Verification items for the finished model (mm, model axes). Face numbers are marked on the shaded views. A direction names the side the tool comes from. Give positions to 0.01 mm unless a question says otherwise; leave off trailing zeros. Write each loop counter-clockwise with the first axis right and the second up, starting at its lowest first coordinate (ties: lowest second). Pieces come first, ordered by that corner, then holes.
from build123d import *

# Parameters (mm, degrees)
F0_R     = 6.5
F1_DEPTH = 8
F3_DEPTH = 4
F4_R     = 4
F5_DEPTH = 45
F6_R     = 4
F6_R_2   = 3.4
F7_DEPTH = 28
F8_SIZE  = 1


with BuildPart() as f1:
    # F0 (on Front) → F1 (new body)
    with BuildSketch(Plane.XZ):
        Circle(F0_R)
    extrude(amount=-F1_DEPTH)

    # F2 (on face) → F3 (cut)
    with BuildSketch(Plane.XZ):
        Polygon((3, 1.732051), (0, 3.464102), (-3, 1.732051), (-3, -1.732051), (0, -3.464102), (3, -1.732051), align=None)
    extrude(amount=-F3_DEPTH, mode=Mode.SUBTRACT)

    # F4 (on face) → F5 (join)
    with BuildSketch(Plane(origin=(0, 8, 0), x_dir=(-1, 0, 0), z_dir=(0, 1, 0))):
        Circle(F4_R)
    extrude(amount=F5_DEPTH)

    # F6 (on face) → F7 (cut)
    with BuildSketch(Plane(origin=(0, 53, 0), x_dir=(-1, 0, 0), z_dir=(0, 1, 0))):
        Circle(F6_R)
        Circle(F6_R_2, mode=Mode.SUBTRACT)
    extrude(amount=-F7_DEPTH, mode=Mode.SUBTRACT)

    # F8
    f8_edges = [f1.edges().sort_by_distance(p)[0] for p in [
        (-6.5, 0, 0),
    ]]
    chamfer(f8_edges, length=F8_SIZE)


solid = f1.part
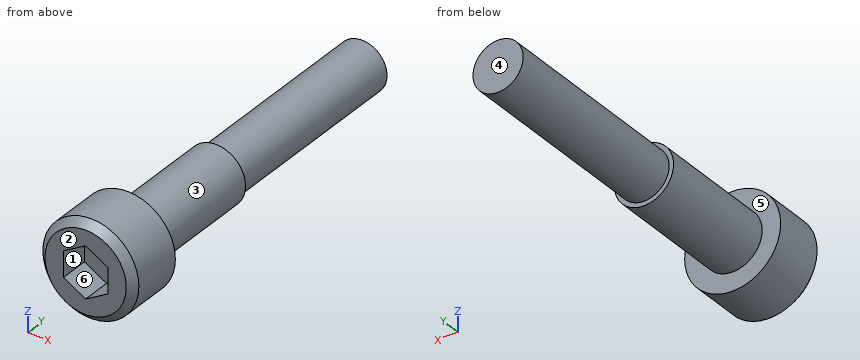
Item 1: Sectioned sample at B-B on z = 0. Record the cut outline in (x, y), then the cut area to 3 significant figures.
Answer key:
outline: (-6.5, 1) - (-5.5, 0) - (-3, 0) - (-3, 4) - (3, 4) - (3, 0) - (5.5, 0) - (6.5, 1) - (6.5, 8) - (4, 8) - (4, 25) - (3.4, 25) - (3.4, 53) - (-3.4, 53) - (-3.4, 25) - (-4, 25) - (-4, 8) - (-6.5, 8) - close
area: 405 mm2
Item 2: Set-up check for the marked faces 4, 5 and 6: record each of +Z, -Z, +X, -X, +Y, -Y from which the full face is reachable in a straight line by a thin tool's end or side.
Answer key:
face 4: +Z, -Z, +X, -X, +Y
face 5: +Y
face 6: -Y
Item 3: Sectioned sample at C-C on y = 48. Record the cut outline in (x, z).
Answer key:
outline: circle Ø6.8 at (0, 0)
Item 4: Release check for a two-part mould opening along X. For the marked faces 1, 2 and 3 record: released by +X, released by -X, zero draft, split by the parting line, or undercut.
Answer key:
face 1: undercut
face 2: zero draft
face 3: split by the parting line
Item 5: Scan lines: line 1 along Y through (x, z) = (-3.5, 0); line 2 along X through (y, z) = (16.5, -0.25); line 3 along X through (y, z) = (20, -2). Record each from-to range of solid material in increasing order.
Answer key:
line 1: y = 0 to 25
line 2: x = -3.99 to 3.99
line 3: x = -3.46 to 3.46
Item 6: Depth check by flat-ended pin: pin 1 (3 mm diameter, centred on x = 1.5, y = 29, fed in from +Z); pin 2 (6 mm diameter, centred on x = 1.5, y = 12, fed in from +Z); pin 3 (4 mm diameter, centred on x = 1.5, y = 23.5, fed in from -Z). Enter the tip coordinate at first touch or a pass-through.
Answer key:
pin 1: stops at z = 3.4
pin 2: stops at z = 4
pin 3: stops at z = -4
Item 7: Sectioned sample at A-A on y = 3. Record the cut outline in (x, z), then the cut area to 3 significant figures.
Answer key:
outline: circle Ø13 at (0, 0); hole (-3, -1.73) - (0, -3.46) - (3, -1.73) - (3, 1.73) - (0, 3.46) - (-3, 1.73) - close
area: 102 mm2
